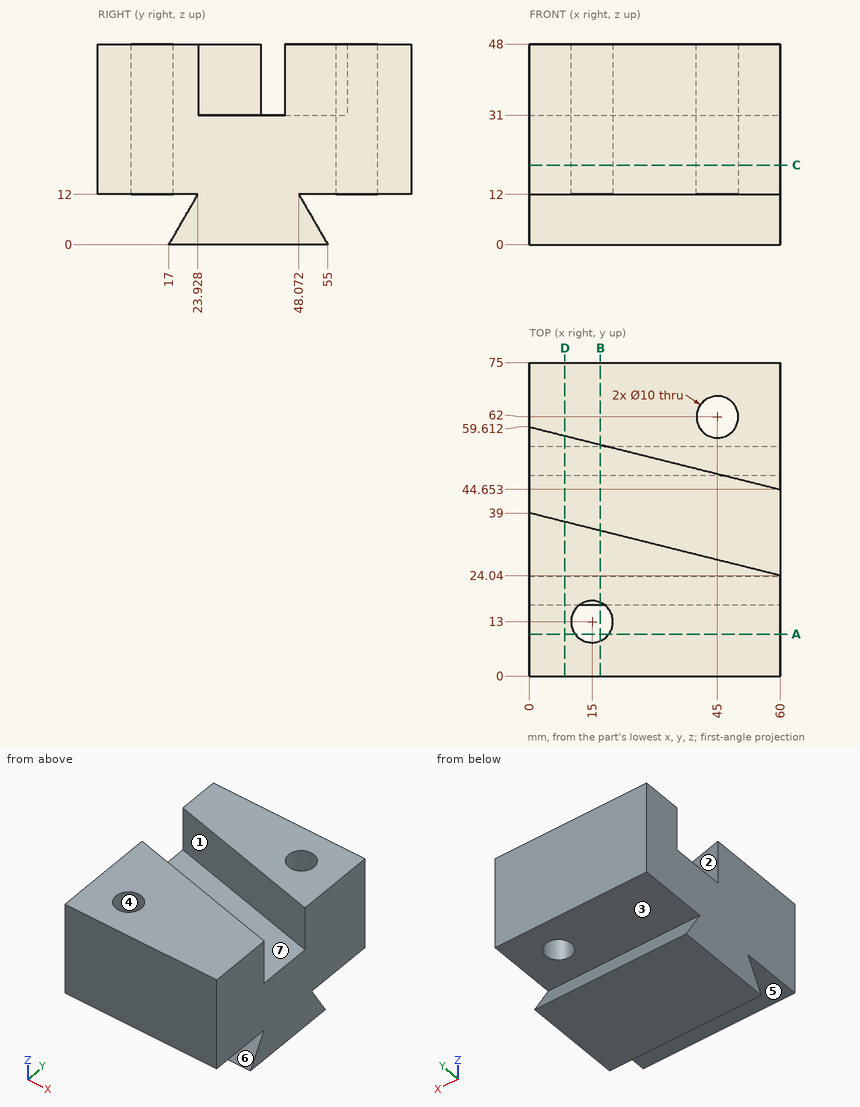
Check sheet for the drawn part. Datum: minimum x, y, z corner. Units: mm. A direction names the side the tool comes from. Round coordinates to 2 decimals unless told otherwise and drop trailing zeros. Order: outer loops, then holes, each group sorted by start corner. A loop starts at its lowest first (then second) coordinate and runs counter-clockwise, first axis right, second up. Notation, with made-up numbers: M 29,62.25 L 77,62.25 A29 cw 77,90.25 Z; hole C -5,79.5 d5. An arc over 180 degrees is marked long. Write each question's results on one line, items separated by ' | '. Start each with the question number.
1. Cross-section at C-C on z = 19. Record the boundary of the cut face in (x, y).
2. Cross-section at A-A on y = 10. Record the boundary of the cut face in (x, z).
3. Go/stop test with flat-tipped pins: P1, Ø8, axis at x = 28, z = 6.5, coming from the -Y side; P2, Ø11.5, axis at x = 45, y = 62, coming from the -Z side. Record where each tip stops, or that it passes through.
4. Material ranges on L1, parallel to X at y = 9, z = 38.5; L2, parallel to Y at x = 45, z = 26; L3, parallel to Y at x = 15, z = 41.5, recorded low to high. Write a range as from..to.
5. Cross-section at D-D on x = 8.5. Record the boundary of the cut face in (y, z), plus the area to 3 significant figures.
6. Draft check along Y on the marked faces 5, 6 and 7. Enter one of: pulls with the +Y half, pulls with the -Y half, needs draft (parallel to the pull), parting line crosses it, or undercut.
7. Set-up check for the marked faces 1, 2, 3 and 4: record each of +Z, -Z, +X, -X, +Y, -Y from which the full face is reachable in a straight line by a thin tool's end or side.
8. Cross-section at B-B on x = 17. Record the boundary of the cut face in (y, z).
Resolved:
1) outline: M 0,0 L 60,0 L 60,75 L 0,75 Z; hole C 15,13 d10; hole C 45,62 d10
2) outline: M 0,12 L 11,12 L 11,48 L 0,48 Z; M 19,12 L 60,12 L 60,48 L 19,48 Z
3) P1: y = 18.44 | P2: z = 12
4) L1: 0..12, 18..60 | L2: 0..57, 67..75 | L3: 0..8, 18..35.26, 55.87..75
5) outline: M 0,12 L 23.93,12 L 17,0 L 55,0 L 48.07,12 L 75,12 L 75,48 L 57.49,48 L 57.49,31 L 36.88,31 L 36.88,48 L 0,48 Z | area: 2,720 mm2
6) face 5: needs draft | face 6: pulls with the -Y half | face 7: undercut
7) face 1: +Z, -X | face 2: +Z, +X | face 3: +X, -X, +Y | face 4: +Z
8) outline: M 0,12 L 8.42,12 L 8.42,48 L 0,48 Z; M 17,0 L 55,0 L 48.07,12 L 75,12 L 75,48 L 55.37,48 L 55.37,31 L 34.76,31 L 34.76,48 L 17.58,48 L 17.58,12 L 23.93,12 Z
